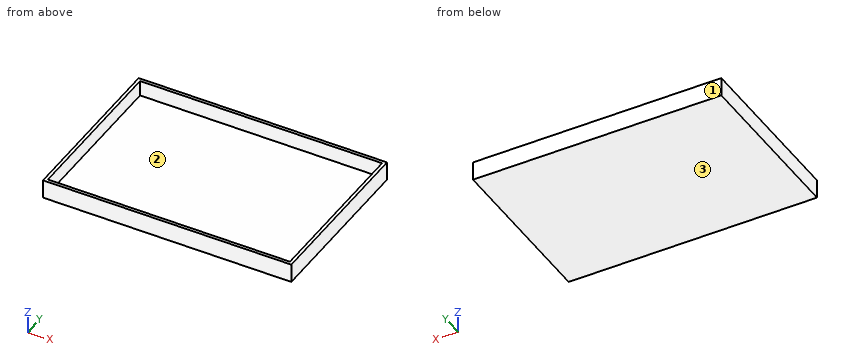
```python
from build123d import *

# Parameters (mm, degrees)
F0_W     = 154
F0_H     = 104
F1_DEPTH = 10
F2_T     = 2


with BuildPart() as f1:
    # F0 (on Top) → F1 (new body)
    with BuildSketch(Plane.XY):
        Rectangle(F0_W, F0_H)
    extrude(amount=F1_DEPTH)

    # F2
    f2_openings = [f1.faces().sort_by_distance(p)[0] for p in [
        (0, 0, 10),
    ]]
    offset(amount=F2_T, openings=f2_openings, kind=Kind.INTERSECTION)


solid = f1.part
```
The model under review builds one solid part; all positions refer to its coordinate system, in mm. Face numbers are marked on the shaded views. Give positions to 0.01 mm unless a question says otherwise; leave off trailing zeros. Write each loop counter-clockwise with the first axis right and the second up, starting at its lowest first coordinate (ties: lowest second). Pieces come first, ordered by that corner, then holes. Notation, with made-up numbers: (24.5, 10) -> (69.5, 10) arc R14 cw to (69.5, 31) -> close; hole circle Ø3 at (42, 68.5). An arc over 180 degrees is marked (long way). Put each result on its own line as item: value.
(1) We need section C-C, the plane y = 41.5. Give the boundary of the cut face in (x, z).
Results are:
outline: (-79, -2) -> (79, -2) -> (79, 10) -> (77, 10) -> (77, 0) -> (-77, 0) -> (-77, 10) -> (-79, 10) -> close
(2) The part is to be moulded in two halves that separate along Y. For the marked faces 1, 2 and 3, say which applies: pulls with the +Y half, pulls with the -Y half, needs draft (parallel to the pull), parting line crosses it, or undercut.
Results are:
face 1: pulls with the +Y half
face 2: undercut
face 3: needs draft
(3) We need section B-B, the plane x = -4.5. Give the boundary of the cut face in (y, z).
Results are:
outline: (-54, -2) -> (54, -2) -> (54, 10) -> (52, 10) -> (52, 0) -> (-52, 0) -> (-52, 10) -> (-54, 10) -> close
(4) To check wall thickness, follow probe 1 along Y at (x, z) = (-13, 9); probe 2 along X at (y, z) = (37, 1.25); probe 3 along Z at (x, y) = (30, 6.5). State the ranges of each line that lie inside material, in increasing order. Write a range as from..to.
Results are:
probe 1: -54..-52, 52..54
probe 2: -79..-77, 77..79
probe 3: -2..0
(5) For pin 1 Ø1 at (x, y) = (-50.5, -37.5) entering from +Z, flat-tipped, find the tip position at first contact; note if it passes through.
Results are:
pin 1: z = 0
(6) We need section A-A, the plane z = 5.5. Give the boundary of the cut face in (x, y), and give its area (3 significant figures).
Results are:
outline: (-79, -54) -> (79, -54) -> (79, 54) -> (-79, 54) -> close; hole (-77, -52) -> (77, -52) -> (77, 52) -> (-77, 52) -> close
area: 1,050 mm²
